Input: part model. Units: mm. Frame: model coordinates. A direction names the side the tool comes from. Coordinates: 2 decimals unless noted, no trailing zeros. Order: outer loops, then holes, each group sorted by start corner. A loop starts at its lowest first (then second) coordinate and runs counter-clockwise, first axis right, second up. Notation, with made-up numbers: M -31.75,-9.5 L 27.25,-9.5 A17 ccw 27.25,5.5 Z; hole C 45.5,-2 d7. An arc over 180 degrees is marked long. One line per item, written item: value.
```python
from build123d import *

# Parameters (mm, degrees)
BOSS_EXTRUDE1_DEPTH = 25
SKETCH4_W           = 80
SKETCH4_H           = 30
SKETCH4_R           = 2.651056997
BOSS_EXTRUDE4_DEPTH = 10


with BuildPart() as part:
    # Sketch1 → Boss-Extrude1 (new body)
    with BuildSketch(Plane(origin=(0, 0, 0), x_dir=(1, 0, 0), z_dir=(0, 1, 0))):
        with BuildLine():
            Line((18.424541272, -35.177357689), (23.005994318, -14.800530945))
            ThreePointArc((23.005994318, -14.800530945), (20.864784183, 0.157407238), (9.326512498, 9.914096331))
            Line((9.326512498, 9.914096331), (9.326512498, 11.603851187))
            Line((9.326512498, 11.603851187), (26.937532501, 11.267061467))
            Line((26.937532501, 11.267061467), (25.932986747, -41.261487659))
            ThreePointArc((25.932986747, -41.261487659), (15.860542773, -43.070975474), (10.227869895, -34.526891555))
            Line((10.227869895, -34.526891555), (10.227869895, -4.048540158))
            ThreePointArc((10.227869895, -4.048540158), (14.304101202, -7.422369294), (15.833057178, -12.488006305))
            Line((15.833057178, -12.488006305), (15.833057178, -33.589930418))
            ThreePointArc((15.833057178, -33.589930418), (16.997270485, -34.598365473), (18.424541272, -35.177357689))
        make_face()
    extrude(amount=BOSS_EXTRUDE1_DEPTH)

    # Sketch4 → Boss-Extrude4 (add)
    with BuildSketch(Plane(origin=(26.712294191, 0, 0.510840717), x_dir=(0.0191203094367821, 0, -0.9998171901738045), z_dir=(0.9998171901738045, 0, 0.0191203094367821))):
        with Locations((-15.719944306, 12.3)):
            Rectangle(SKETCH4_W, SKETCH4_H)
        with Locations((-50.219944306, 12.3)):
            Circle(SKETCH4_R, mode=Mode.SUBTRACT)
        with Locations((18.780055694, 12.3)):
            Circle(SKETCH4_R, mode=Mode.SUBTRACT)
    extrude(amount=BOSS_EXTRUDE4_DEPTH)


solid = part.part
```
(1) Draft query along Z for faces 6 (the flat face through (14, 0, 16)), 7 (the cylindrical face through (30.631, 12.417, 53.464)). Return one class per face: released by +Z, released by -Z, zero draft, split by the parting line, or undercut.
Data:
face 6: zero draft
face 7: undercut
(2) Cut plane B-B on y = 11. Output: boundary loops of the cut face in (x, z), plus the area to 3 significant figures.
Data:
outline: M 9.33,-11.6 L 26.94,-11.27 L 27.03,-15.96 L 37.03,-15.76 L 35.79,48.6 L 25.8,48.41 L 25.93,41.26 A9.3 ccw 10.23,34.53 L 10.23,4.05 A9.16 ccw 15.83,12.49 L 15.83,33.59 A4.71 cw 18.42,35.18 L 23.01,14.8 A21.26 cw 9.33,-9.91 Z; M 25.65,56.22 L 25.71,53.03 L 35.71,53.22 L 35.65,56.41 Z; M 27.12,-20.58 L 27.18,-23.76 L 37.17,-23.57 L 37.11,-20.38 Z
area: 1,280 mm2
(3) Access query for faces 1 (the flat face through (31, 27.3, 17)), 2 (the flat face through (10.228, 12, 20)), 3 (the cylindrical face through (32, 13.1, -20.7)), 4 (the flat face through (15.833, 12, 23)), 5 (the flat face through (14, 25, 16)). Directions: +Z, -Z, +X, -X, +Y, -Y. A direction counts if a zero-diameter tool reaches every point of the face in a straight line with its end or side. Return the directions, or none.
Data:
face 1: +Z, -Z, +X, -X, +Y
face 2: +Z, -X, +Y, -Y
face 3: none
face 4: +Y, -Y
face 5: -Z, -X, +Y
(4) Cut plane A-A on z = 9. Output: boundary loops of the cut face in (x, y), plus the area to 3 significant figures.
Data:
outline: M 10.23,0 L 15.14,0 L 15.14,25 L 10.23,25 Z; M 23.49,0 L 26.55,0 L 26.55,-2.7 L 36.55,-2.7 L 36.55,27.3 L 26.55,27.3 L 26.55,25 L 23.49,25 Z
area: 499 mm2
(5) Cut plane C-C on x = 19.5. Output: boundary loops of the cut face in (y, z), plus the area to 3 significant figures.
Data:
outline: M 0,-11.41 L 25,-11.41 L 25,-2.31 L 0,-2.31 Z; M 0,30.39 L 25,30.39 L 25,43.82 L 0,43.82 Z
area: 563 mm2
(6) Ray query, line 1 (Z direction, x = 30.5, y = 12.75); line 2 (Y direction, x = 34.5, z = 50); line 3 (Y direction, x = 24, z = 7.5). Return the intervals inside material, ascending. Write a range as from..to.
Data:
line 1: z = -23.7..-20.81, -15.59..48.2, 53.43..56.31
line 2: y = -2.7..9.8, 14.8..27.3
line 3: y = 0..25
(7) Cut plane D-D on z = 42. Output: boundary loops of the cut face in (x, y), plus the area to 3 significant figures.
Data:
outline: M 13.99,0 L 25.05,0 L 25.05,25 L 13.99,25 Z; M 25.92,-2.7 L 35.92,-2.7 L 35.92,27.3 L 25.92,27.3 Z
area: 577 mm2
(8) First-contact query: pin 1 (5 mm diameter, centred on y = 10.5, z = 48, fed in from -X); pin 2 (10 mm diameter, centred on x = 33, y = 15, fed in from +Z); pin 3 (1.5 mm diameter, centred on y = 11.5, z = -2.5, fed in from +X); pin 4 (8 mm diameter, centred on y = 2.5, z = 8, fed in from -X). Flat tips, straight axial feed; report the tip coordinate or a pass-through.
Data:
pin 1: stops at x = 25.76
pin 2: stops at z = 56.41
pin 3: stops at x = 36.79
pin 4: stops at x = 10.23
